from build123d import *

# Parameters (mm, degrees)
SKETCH1_W                      = 25.4
SKETCH1_H                      = 152.4
BOSS_EXTRUDE1_DEPTH            = 25.4
SKETCH2_W                      = 22.225
SKETCH2_H                      = 22.225
CUT_EXTRUDE1_DEPTH             = 279.4
F_3_16_0_1875_DIAMETER_HOLE2_D = 4.7625
F_1_8_0_125_DIAMETER_HOLE1_D   = 3.175


with BuildPart() as part:
    # Sketch1 → Boss-Extrude1 (new body)
    with BuildSketch(Plane.XY):
        with Locations((76.086049872, -101.14964539)):
            Rectangle(SKETCH1_W, SKETCH1_H)
    extrude(amount=BOSS_EXTRUDE1_DEPTH)

    # Sketch2 → Cut-Extrude1 (cut)
    with BuildSketch(Plane(origin=(0, -24.94964539, 0), x_dir=(1, 0, 0), z_dir=(0, 1, 0))):
        with Locations((76.086049872, -12.7)):
            Rectangle(SKETCH2_W, SKETCH2_H)
    extrude(amount=-CUT_EXTRUDE1_DEPTH, mode=Mode.SUBTRACT)

    # 3/16 (0.1875) Diameter Hole2 (through all)
    with Locations(Plane(origin=(88.786049872, 0, 0), x_dir=(0, 0, -1), z_dir=(1, 0, 0))):
        with Locations((-19.05, -173.53964539), (-19.05, -28.75964539)):
            Hole(F_3_16_0_1875_DIAMETER_HOLE2_D / 2)

    # 1/8 (0.125) Diameter Hole1 (through all)
    with Locations(Plane(origin=(88.786049872, 0, 0), x_dir=(0, 0, -1), z_dir=(1, 0, 0))):
        with Locations((-21.59, -77.01964539), (-8.89, -77.01964539), (-21.59, -54.15964539), (-8.89, -54.15964539)):
            Hole(F_1_8_0_125_DIAMETER_HOLE1_D / 2)


solid = part.part
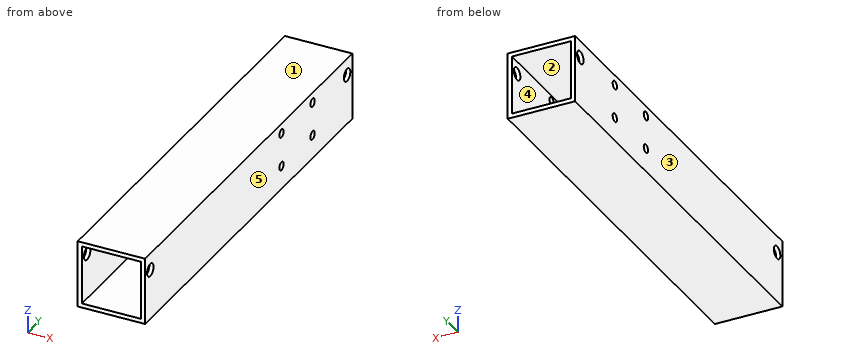
Geometry check sheet. Reference: the model listing, model coordinates, mm. Face numbers are marked on the shaded views. A direction names the side the tool comes from. Give positions to 0.01 mm unless a question says otherwise; leave off trailing zeros. Order: outer loops, then holes, each group sorted by start corner. A loop starts at its lowest first (then second) coordinate and runs counter-clockwise, first axis right, second up.
1. Sectioned sample at A-A (z = 12). Record the boundary of the cut face in (x, y), then the cut area to 3 significant figures.
Completed:
outline: (63.39, -177.35) - (64.97, -177.35) - (64.97, -24.95) - (63.39, -24.95) - close; (87.2, -177.35) - (88.79, -177.35) - (88.79, -24.95) - (87.2, -24.95) - close
area: 484 mm2
2. Draft check along X on the marked faces 1, 2 and 3. Enter one of: pulls with the +X half, pulls with the -X half, needs draft (parallel to the pull), parting line crosses it, or undercut.
Completed:
face 1: needs draft
face 2: undercut
face 3: pulls with the -X half
3. Depth check by flat-ended pin: pin 1 (3 mm diameter, centred on y = -77.02, z = 8.89, fed in from +X). Enter the tip coordinate at first touch or a pass-through.
Completed:
pin 1: passes through
4. Sectioned sample at C-C (y = -51). Record the boundary of the cut face in (x, z), then the cut area to 3 significant figures.
Completed:
outline: (63.39, 0) - (88.79, 0) - (88.79, 25.4) - (63.39, 25.4) - close; hole (64.97, 1.59) - (87.2, 1.59) - (87.2, 23.81) - (64.97, 23.81) - close
area: 151 mm2
5. Sectioned sample at B-B (x = 83.25). Record the boundary of the cut face in (y, z).
Completed:
outline: (-177.35, 0) - (-24.95, 0) - (-24.95, 1.59) - (-177.35, 1.59) - close; (-177.35, 23.81) - (-24.95, 23.81) - (-24.95, 25.4) - (-177.35, 25.4) - close
6. Scan lines: line 1 (Y direction, x = 64.6, z = 8.89); line 2 (Y direction, x = 64.1, z = 19.05); line 3 (X direction, y = -93, z = 11.5). Record each from-to range of solid material in increasing order.
Completed:
line 1: y = -177.35 to -78.61, -75.43 to -55.75, -52.57 to -24.95
line 2: y = -177.35 to -175.92, -171.16 to -31.14, -26.38 to -24.95
line 3: x = 63.39 to 64.97, 87.2 to 88.79
7. Access from +Z, -Z, +X, -X, +Y, -Y to the whole of each face (thin tool, end or side, straight path). Record for the marked faces 4 and 5.
Completed:
face 4: +Y, -Y
face 5: +Z, -Z, +X, +Y, -Y
